Part model, mm, in its own coordinate system. A direction names the side the tool comes from. Give positions to 0.01 mm unless a question says otherwise; leave off trailing zeros. Order: outer loops, then holes, each group sorted by start corner. A loop starts at its lowest first (then second) coordinate and runs counter-clockwise, first axis right, second up. Notation, with made-up numbers: M 56,66 L 83,66 A33 ccw 83,97 Z; hole C -31.75,38.25 d8. An arc over 180 degrees is marked long. Return JSON: item names as keys, results as strings.
Autodesk Inventor part; units mm, degrees
ref_plane "YZ Plane" through (0, 0, 0) normal (1, 0, 0) x (0, 1, 0)
ref_plane "XZ Plane" through (0, 0, 0) normal (0, 1, 0) x (-1, 0, 0)
ref_plane "XY Plane" through (0, 0, 0) normal (0, 0, 1) x (1, 0, 0)
sketch "スケッチ1" plane through (0, 0, 0) normal (0, 1, 0) x (-1, 0, 0)
  line L0 (0, 0) -> (-64.0652, 0) construction
  circle A0 centre (-31.65, 0) radius 2.85
  line L1 (-26.65, -3.5) -> (-31.65, -3.5)
  line L2 (-31.65, -3.5) -> (-31.65, 3.5)
  line L3 (-31.65, 3.5) -> (-26.65, 3.5)
  line L4 (-26.65, 3.5) -> (-26.65, -3.5)
  line L5 (0, -4.9) -> (0, 4.9)
  point P0 (-31.65, 2.85)
  point P1 (-31.65, -2.85)
  dimension "P_DIA" = 5.7
  dimension "P_D1" = 31.65
  dimension "d2" = 7
  dimension "d3" = 5
revolve "リム" add sketch "スケッチ1" angle 360 about axis through (0, 0, -10) along (0, 0, 1) contours A0 L2 L3 L4 L1
sketch "スケッチ3" plane through (0, 0, 3.5) normal (0, 0, 1) x (1, 0, 0)
  line L0 (-5, 2.8868) -> (0, 5.7735)
  line L1 (0, 5.7735) -> (5, 2.8868)
  line L2 (5, 2.8868) -> (5, -2.8868)
  line L3 (5, -2.8868) -> (0, -5.7735)
  line L4 (0, -5.7735) -> (-5, -2.8868)
  line L5 (-5, -2.8868) -> (-5, 2.8868)
  point P0 (0, 0)
  point P1 (0, 0)
  dimension "HUB_DIA" = 10
extrude "ハブ" add sketch "スケッチ3" against normal up to surface (7 mm away)
sketch "スケッチ4" plane through (0, 0, 3.5) normal (0, 0, 1) x (1, 0, 0)
  line L0 (-0.8, 0) -> (0.8, 0)
  line L1 (0.8, 0) -> (0.8, 26.65)
  line L2 (0.8, 26.65) -> (-0.8, 26.65)
  line L3 (-0.8, 26.65) -> (-0.8, 0)
  circle A0 centre (0, 0) radius 26.65
  point P0 (0, 26.65)
  dimension "SPOKE_THIN" = 1.6
extrude "スポーク" add sketch "スケッチ4" against normal up to surface (7 mm away) contours L3 A0 L1 L0 | L3 L2 A0 | A0 L2 L1 picked at (0, 8.8833)
pattern_circular "円形状パターン1" count 6 over 360 about axis through (0, 0, -10) along (0, 0, 1) of "スポーク"
sketch "スケッチ5" plane through (0, 0, 3.5) normal (0, 0, 1) x (1, 0, 0)
  line L0 (-2.5, 1.525) -> (2.5, 1.525)
  line L1 (2.5, 1.525) -> (2.5, -1.525)
  line L2 (2.5, -1.525) -> (-2.5, -1.525)
  line L3 (-2.5, -1.525) -> (-2.5, 1.525)
  point P0 (0, 0)
  point P1 (0, 1.525)
  point P2 (-2.5, 0)
  dimension "d15" = 5
  dimension "d16" = 3.05
extrude "軸穴" cut sketch "スケッチ5" against normal through all
equation "\"P_D1\" = 0.5 * INNER_DIA + 0.5 * P_DIA"
equation "\"INNER_DIA\" = 57.6"
properties part number "Wheel-D69C"
Q1. Band-saw the part on C-C (z = -0.5). Give the number of separate pieces and of enclosed holes in the cut face, then the cut area to 3 significant figures.
Established:
{"separate pieces": "1", "enclosed holes": "7", "area": "656 mm²"}
Q2. 3-axis set-ups, long thin cutter, end or side, ignore diameter. For faces 4 (the flat face through (-5, 0, 0)), 5 (the flat face through (2, -2, 3.5)): which of +Z, -Z, +X, -X, +Y, -Y reach the whole face in a straight line?
Established:
{"face 4": "+Z, -Z", "face 5": "+Z, +X, -X, +Y, -Y"}
Q3. Band-saw the part on B-B (x = 0). Give the cut face in (y, z) (3 decimals).
Established:
{"outline": "M -31.65,-3.5 L -1.525,-3.5 L -1.525,3.5 L -31.65,3.5 L -31.65,2.85 A2.85 cw -31.65,-2.85 Z; M 1.525,-3.5 L 31.65,-3.5 L 31.65,-2.85 A2.85 cw 31.65,2.85 L 31.65,3.5 L 1.525,3.5 Z"}
Q4. Probe line 1 along Y through (x, z) = (-7.5, -2); line 2 along X through (y, z) = (3, -3); line 3 along X through (y, z) = (5.5, 1.5). List the from-to ranges inside material, lowest first.
Established:
{"line 1": "y = -28.65 to -25.57, -5.25 to -3.41, 3.41 to 5.25, 25.57 to 28.65", "line 2": "x = -31.51 to -26.48, -6.8 to 6.8, 26.48 to 31.51", "line 3": "x = -28.7 to -26.08, -11.13 to -7.93, -0.8 to 0.8, 7.93 to 11.13, 26.08 to 28.7"}
Q5. Band-saw the part on A-A (y = 0). Give the cut face in (x, z), then the cut area to 3 significant figures.
Established:
{"outline": "M -31.65,-3.5 L -26.65,-3.5 L -26.65,3.5 L -31.65,3.5 L -31.65,2.85 A2.85 cw -31.65,-2.85 Z; M -5,-3.5 L -2.5,-3.5 L -2.5,3.5 L -5,3.5 Z; M 2.5,-3.5 L 5,-3.5 L 5,3.5 L 2.5,3.5 Z; M 26.65,-3.5 L 31.65,-3.5 L 31.65,-2.85 A2.85 cw 31.65,2.85 L 31.65,3.5 L 26.65,3.5 Z", "area": "79.5 mm²"}
Q6. Two-plate mould, pull along Y, no slides. Class faces 1 (the cylindrical face through (-6.861, -30.897, 3.18)), 2 (the cylindrical face through (13.17, 23.17, -0.05)), 3 (the flat face through (2, -2, -3.5)): +Y half, -Y half, draft (parallel to the pull), parting line (faces both ways), or undercut.
Established:
{"face 1": "parting line", "face 2": "undercut", "face 3": "draft"}
Q7. Pin check, flat tips, straight feed: pin 1 (2.5 mm diameter, centred on y = 0, z = -1, fed in from +X); pin 2 (2 mm diameter, centred on y = 1, z = -1.5, fed in from -X); pin 3 (1 mm diameter, centred on x = 4, z = -1.5, fed in from +Y). Stop position of each tip, or through.
Established:
{"pin 1": "stops at x = 29.9", "pin 2": "stops at x = -30.27", "pin 3": "stops at y = 29.35"}
